```python
from build123d import *

# Parameters (mm, degrees)
SKETCH1_R           = 1.5
BOSS_EXTRUDE2_DEPTH = 12
SKETCH3_W           = 1.5
SKETCH3_H           = 9
CUT_EXTRUDE2_DEPTH  = 24.832750576
SKETCH4_R           = 1.05
CUT_EXTRUDE3_DEPTH  = 37.510272527
FILLET1_START       = -1
FILLET1_DEPTH       = 14
FILLET1_2_DEPTH     = 12
FILLET1_3_DEPTH     = 1.5
FILLET1_START_2     = 10.5
FILLET1_4_DEPTH     = 1.5


with BuildPart() as part:
    # Sketch1 → Boss-Extrude2 (new body)
    with BuildSketch(Plane.XY):
        with BuildLine():
            ThreePointArc((-10, 0), (-8.5, -1.5), (-7, 0))
            Line((-7, 0), (-10, 0))
        make_face()
        with BuildLine():
            Line((-10, 0), (-7, 0))
            ThreePointArc((-7, 0), (-8.5, 1.5), (-10, 0))
        make_face()
        Polygon((3, 15), (3, 1.5), (3, 0), (6, 0), (6, 15), align=None)
        with BuildLine():
            Line((0, 27), (0, 1.5))
            ThreePointArc((0, 1.5), (1.5, 3), (3, 1.5))
            Line((3, 1.5), (3, 15))
            Line((3, 15), (3, 30))
            ThreePointArc((3, 30), (2.121320344, 32.121320344), (0, 33))
            Line((0, 33), (-7, 33))
            ThreePointArc((-7, 33), (-9.121320344, 32.121320344), (-10, 30))
            Line((-10, 30), (-10, 0))
            ThreePointArc((-10, 0), (-8.5, 1.5), (-7, 0))
            Line((-7, 0), (-7, 27))
            ThreePointArc((-7, 27), (-6.121320344, 29.121320344), (-4, 30))
            Line((-4, 30), (-3, 30))
            ThreePointArc((-3, 30), (-0.878679656, 29.121320344), (0, 27))
        make_face()
        with Locations((1.5, 1.5)):
            Circle(SKETCH1_R)
        with BuildLine():
            ThreePointArc((3, 1.5), (2.560660172, 0.439339828), (1.5, 0))
            Line((1.5, 0), (3, 0))
            Line((3, 0), (3, 1.5))
        make_face()
    extrude(amount=BOSS_EXTRUDE2_DEPTH)

    # Sketch3 → Cut-Extrude2 (cut, through all)
    with BuildSketch(Plane(origin=(0, 15, 0), x_dir=(1, 0, 0), z_dir=(0, 1, 0))):
        with Locations((4.5, -6)):
            Rectangle(SKETCH3_W, SKETCH3_H)
    extrude(amount=-CUT_EXTRUDE2_DEPTH, mode=Mode.SUBTRACT)

    # Sketch4 → Cut-Extrude3 (cut, through all)
    with BuildSketch(Plane.XY.offset(12)):
        with Locations((4.5, 7.5)):
            Circle(SKETCH4_R)
    extrude(amount=-CUT_EXTRUDE3_DEPTH, mode=Mode.SUBTRACT)

    # Fillet1: read off the stored shape, not the designer's step
    # Fillet1 outline → Fillet1 (cut)
    with BuildSketch(Plane.XY.offset(FILLET1_START)):
        with BuildLine():
            Line((6, 14), (6, 15))
            Line((6, 15), (5, 15))
            ThreePointArc((5, 15), (5.707106781, 14.707106781), (6, 14))
        make_face()
    extrude(amount=FILLET1_DEPTH, mode=Mode.SUBTRACT)

    # Fillet1 2 outline → Fillet1 2 (add)
    with BuildSketch(Plane.XY):
        with BuildLine():
            Line((3.75, 15), (3.75, 15.031754164))
            ThreePointArc((3.75, 15.031754164), (3.209430585, 15.387627564), (3, 16))
            Line((3, 16), (3, 15))
            Line((3, 15), (3.75, 15))
        make_face()
    extrude(amount=FILLET1_2_DEPTH)

    # Fillet1 3 outline → Fillet1 3 (add)
    with BuildSketch(Plane.XY):
        with BuildLine():
            Line((3.75, 15), (4, 15))
            ThreePointArc((4, 15), (3.873995708, 15.007970304), (3.75, 15.031754164))
            Line((3.75, 15.031754164), (3.75, 15))
        make_face()
    extrude(amount=FILLET1_3_DEPTH)

    # Fillet1 4 outline → Fillet1 4 (add)
    with BuildSketch(Plane.XY.offset(FILLET1_START_2)):
        with BuildLine():
            Line((3.75, 15), (4, 15))
            ThreePointArc((4, 15), (3.873995708, 15.007970304), (3.75, 15.031754164))
            Line((3.75, 15.031754164), (3.75, 15))
        make_face()
    extrude(amount=FILLET1_4_DEPTH)


solid = part.part
```
Part model, mm, in its own coordinate system. A direction names the side the tool comes from. Round coordinates to 2 decimals unless told otherwise and drop trailing zeros. Order: outer loops, then holes, each group sorted by start corner. A loop starts at its lowest first (then second) coordinate and runs counter-clockwise, first axis right, second up. Notation, with made-up numbers: M 26,20.25 L 40,20.25 A12 ccw 40,32.25 Z; hole C 78,4.5 d9. An arc over 180 degrees is marked long. Answer in a Markdown table with one row per item. Add a question column.
Q1. Mould opens along Z. For faces 1 (the face through (3.75, 3, 6)), 2 (the face through (-0.9, 29.14, 5.92)) say: +Z half, -Z half, draft (parallel to the pull), parting line (faces both ways), or undercut.
Q2. Cut at D-D on y = 29. Give the cut face in (x, z), and give its area (3 significant figures).
Q3. 3-axis set-ups, long thin cutter, end or side, ignore diameter. For faces 3 (the face through (-3, 33, 6)), 4 (the face through (3, 0, 6)), 5 (the face through (3, 23, 6)), 6 (the face through (4, 3, 10.5)), 7 (the face through (0.43, 0.45, 5.92)): which of +Z, -Z, +X, -X, +Y, -Y reach the whole face in a straight line?
Q4. Wall check: L1, parallel to X at y = 6, z = 7.5; L2, parallel to X at y = 15, z = 9.25; L3, parallel to X at y = 19, z = 3.5. Give the ranges that are in metal, low to high. Write a range as from..to.
Q5. Pin check, flat tips, straight feed: pin 1 (0.5 mm diameter, centred on x = 4.5, z = 11.5, fed in from +Y); pin 2 (3.5 mm diameter, centred on y = 20, z = 3.5, fed in from +X); pin 3 (3.5 mm diameter, centred on x = 4, z = 6, fed in from -Y); pin 4 (3.5 mm diameter, centred on x = 4.5, y = 7.5, fed in from -Z). Stop position of each tip, or through.
Q6. Cut at A-A on y = 5. Give the cut face in (x, z), and give its area (3 significant figures).
Q7. Cut at B-B on z = 3.25. Give the cut face in (x, y), and give its area (3 significant figures).
Q8. Cut at C-C on z = 1. Give the cut face in (x, y), and give its area (3 significant figures).
Established:
| question | item | result |
|---|---|---|
| 1 | face 1 | undercut |
| 1 | face 2 | draft |
| 2 | outline | M -10,0 L -6.24,0 L -6.24,12 L -10,12 Z; M -0.76,0 L 3,0 L 3,12 L -0.76,12 Z |
| 2 | area | 90.3 mm2 |
| 3 | face 3 | +Z, -Z, +X, -X, +Y |
| 3 | face 4 | +Z, -Z, +X, -Y |
| 3 | face 5 | +Z, -Z, +X, +Y |
| 3 | face 6 | +Y, -Y |
| 3 | face 7 | +Z, -Z, -Y |
| 4 | L1 | x = -10..-7, 0..3.75, 5.25..6 |
| 4 | L2 | x = -10..-7, 0..3.75 |
| 4 | L3 | x = -10..-7, 0..3 |
| 5 | pin 1 | stops at y = 15 |
| 5 | pin 2 | stops at x = 3 |
| 5 | pin 3 | stops at y = 0 |
| 5 | pin 4 | stops at z = 0 |
| 6 | outline | M -10,0 L -7,0 L -7,12 L -10,12 Z; M 0,0 L 6,0 L 6,12 L 0,12 Z; hole M 3.75,1.5 L 5.25,1.5 L 5.25,10.5 L 3.75,10.5 Z |
| 6 | area | 94.5 mm2 |
| 7 | outline | M -10,0 A1.5 ccw -7,0 L -7,27 A3 cw -4,30 L -3,30 A3 cw 0,27 L 0,1.5 A1.5 ccw 1.5,0 L 3.75,0 L 3.75,6.77 A1.05 cw 3.75,8.23 L 3.75,15.03 A1 cw 3,16 L 3,30 A3 ccw 0,33 L -7,33 A3 ccw -10,30 Z; M 5.25,0 L 6,0 L 6,14 A1 ccw 5.25,14.97 L 5.25,8.23 A1.05 cw 5.25,6.77 Z |
| 7 | area | 244 mm2 |
| 8 | outline | M -10,0 A1.5 ccw -7,0 L -7,27 A3 cw -4,30 L -3,30 A3 cw 0,27 L 0,1.5 A1.5 ccw 1.5,0 L 6,0 L 6,14 A1 ccw 5,15 L 4,15 A1 cw 3,16 L 3,30 A3 ccw 0,33 L -7,33 A3 ccw -10,30 Z; hole C 4.5,7.5 d2.1 |
| 8 | area | 264 mm2 |
